from build123d import *

# Parameters (mm, degrees)
CROQUIS1_W              = 16
CROQUIS1_H              = 11.5
SALIENTE_EXTRUIR2_DEPTH = 8
CROQUIS3_W              = 14
CROQUIS3_H              = 9.5
CORTAR_EXTRUIR2_DEPTH   = 2
CROQUIS4_W              = 12
CROQUIS4_H              = 7.5
CORTAR_EXTRUIR3_DEPTH   = 5
REDONDEO1_R             = 1
REDONDEO2_R             = 0.5
CORTAR_EXTRUIR4_REACH   = 19.119
CROQUIS5_R              = 0.5
CORTAR_EXTRUIR5_REACH   = 16.773
CROQUIS6_R              = 0.5


with BuildPart() as part:
    # Croquis1 → Saliente-Extruir2 (new body)
    with BuildSketch(Plane(origin=(0, 0, 0), x_dir=(1, 0, 0), z_dir=(0, 1, 0))):
        Rectangle(CROQUIS1_W, CROQUIS1_H)
    extrude(amount=SALIENTE_EXTRUIR2_DEPTH)

    # Croquis3 → Cortar-Extruir2 (cut)
    with BuildSketch(Plane(origin=(0, 8, 0), x_dir=(1, 0, 0), z_dir=(0, 1, 0))):
        Rectangle(CROQUIS3_W, CROQUIS3_H)
    extrude(amount=-CORTAR_EXTRUIR2_DEPTH, mode=Mode.SUBTRACT)

    # Croquis4 → Cortar-Extruir3 (cut)
    with BuildSketch(Plane(origin=(0, 6, 0), x_dir=(1, 0, 0), z_dir=(0, 1, 0))):
        Rectangle(CROQUIS4_W, CROQUIS4_H)
    extrude(amount=-CORTAR_EXTRUIR3_DEPTH, mode=Mode.SUBTRACT)

    # Redondeo1
    redondeo1_edges = [part.edges().sort_by_distance(p)[0] for p in [
        (0, 0, 5.75),
        (8, 0, 0),
        (0, 0, -5.75),
        (-8, 0, 0),
        (-8, 4, 5.75),
        (8, 4, 5.75),
        (8, 4, -5.75),
        (-8, 4, -5.75),
    ]]
    fillet(redondeo1_edges, radius=REDONDEO1_R)

    # Redondeo2
    redondeo2_edges = [part.edges().sort_by_distance(p)[0] for p in [
        (7, 7, -4.75),
        (7, 7, 4.75),
        (-7, 7, 4.75),
        (-7, 7, -4.75),
    ]]
    fillet(redondeo2_edges, radius=REDONDEO2_R)

    # Croquis5 → Cortar-Extruir4 (cut, up to next)
    with BuildSketch(Plane.ZY.offset(-6), mode=Mode.PRIVATE) as cortar_extruir4_sk1:
        with Locations((-1.27, 3.5)):
            Circle(CROQUIS5_R)
    cortar_extruir4_tool1 = extrude(cortar_extruir4_sk1.sketch, amount=-CORTAR_EXTRUIR4_REACH, mode=Mode.PRIVATE) & part.part
    # Croquis5 → Cortar-Extruir4 (cut, up to next)
    with BuildSketch(Plane.ZY.offset(-6), mode=Mode.PRIVATE) as cortar_extruir4_sk2:
        with Locations((1.27, 3.5)):
            Circle(CROQUIS5_R)
    cortar_extruir4_tool2 = extrude(cortar_extruir4_sk2.sketch, amount=-CORTAR_EXTRUIR4_REACH, mode=Mode.PRIVATE) & part.part
    add(cortar_extruir4_tool1.solids().sort_by_distance((6, 3.5, -1.27))[0], mode=Mode.SUBTRACT)
    add(cortar_extruir4_tool2.solids().sort_by_distance((6, 3.5, 1.27))[0], mode=Mode.SUBTRACT)

    # Croquis6 → Cortar-Extruir5 (cut, up to next)
    with BuildSketch(Plane.XY.offset(-3.75), mode=Mode.PRIVATE) as cortar_extruir5_sk1:
        with Locations((1.905, 3.5)):
            Circle(CROQUIS6_R)
    cortar_extruir5_tool1 = extrude(cortar_extruir5_sk1.sketch, amount=-CORTAR_EXTRUIR5_REACH, mode=Mode.PRIVATE) & part.part
    # Croquis6 → Cortar-Extruir5 (cut, up to next)
    with BuildSketch(Plane.XY.offset(-3.75), mode=Mode.PRIVATE) as cortar_extruir5_sk2:
        with Locations((-1.905, 3.5)):
            Circle(CROQUIS6_R)
    cortar_extruir5_tool2 = extrude(cortar_extruir5_sk2.sketch, amount=-CORTAR_EXTRUIR5_REACH, mode=Mode.PRIVATE) & part.part
    add(cortar_extruir5_tool1.solids().sort_by_distance((1.905, 3.5, -3.75))[0], mode=Mode.SUBTRACT)
    add(cortar_extruir5_tool2.solids().sort_by_distance((-1.905, 3.5, -3.75))[0], mode=Mode.SUBTRACT)


solid = part.part
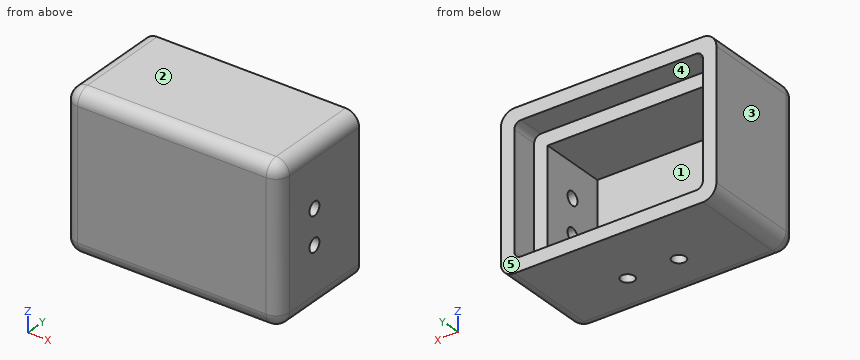
Geometry check sheet. Reference: the model listing, model coordinates, mm. Face numbers are marked on the shaded views. A direction names the side the tool comes from. Give positions to 0.01 mm unless a question says otherwise; leave off trailing zeros. Order: outer loops, then holes, each group sorted by start corner. A loop starts at its lowest first (then second) coordinate and runs counter-clockwise, first axis right, second up. Notation, with made-up numbers: M 74,-26.75 L 93,-26.75 A18 ccw 93,-10.75 Z; hole C -15.5,68 d6. An arc over 180 degrees is marked long. Use a Markdown table: item, result.
Item 1: Section check B-B (y = 1.5). Record the cut outline in (x, z).
Answers follow:
| item | result |
|---|---|
| outline | M -8,-4.75 A1 ccw -7,-5.75 L 7,-5.75 A1 ccw 8,-4.75 L 8,4.75 A1 ccw 7,5.75 L -7,5.75 A1 ccw -8,4.75 Z; hole M -6,-3.75 L 6,-3.75 L 6,3.75 L -6,3.75 Z |
Item 2: Section check D-D (x = -5.75). Record the cut outline in (y, z).
Answers follow:
| item | result |
|---|---|
| outline | M 0,-4.75 A1 ccw 1,-5.75 L 8,-5.75 L 8,-4.75 L 6,-4.75 L 6,-3.75 L 1,-3.75 L 1,3.75 L 6,3.75 L 6,4.75 L 8,4.75 L 8,5.75 L 1,5.75 A1 ccw 0,4.75 Z |
Item 3: Tool access check on the marked faces 1 and 2. Record the directions out of +Z, -Z, +X, -X, +Y, -Y that give a thin tool (end or side, any length) a straight path to the whole face; none if there is none.
Answers follow:
| item | result |
|---|---|
| face 1 | +Y |
| face 2 | +Z, +X, -X, +Y, -Y |
Item 4: Section check A-A (y = 3.5). Record the cut outline in (x, z) (3 decimals).
Answers follow:
| item | result |
|---|---|
| outline | M -8,-4.75 A1 ccw -7,-5.75 L -2.405,-5.75 L -2.405,-3.75 L -6,-3.75 L -6,3.75 L 6,3.75 L 6,1.77 L 8,1.77 L 8,4.75 A1 ccw 7,5.75 L -7,5.75 A1 ccw -8,4.75 Z; M -1.405,-5.75 L 1.405,-5.75 L 1.405,-3.75 L -1.405,-3.75 Z; M 2.405,-5.75 L 7,-5.75 A1 ccw 8,-4.75 L 8,-1.77 L 6,-1.77 L 6,-3.75 L 2.405,-3.75 Z; M 6,-0.77 L 8,-0.77 L 8,0.77 L 6,0.77 Z |
Item 5: Depth check by flat-ended pin: P1, Ø2, axis at x = -0.5, z = 1, coming from the +Y side. Enter the tip coordinate at first touch or a pass-through.
Answers follow:
| item | result |
|---|---|
| P1 | stops at y = 1 |
Item 6: Draft check along X on the marked faces 3, 4 and 5. Enter one of: +X half, -X half, draft (parallel to the pull), parting line (faces both ways), or undercut.
Answers follow:
| item | result |
|---|---|
| face 3 | -X half |
| face 4 | undercut |
| face 5 | draft |
Item 7: Material ranges on line 1 along Z through (x, y) = (-1, 4.25); line 2 along X through (y, z) = (3, 3); line 3 along X through (y, z) = (6.25, 3), recorded low to high.
Answers follow:
| item | result |
|---|---|
| line 1 | z = -5.75 to -3.75, 3.75 to 5.75 |
| line 2 | x = -8 to -6, 6 to 8 |
| line 3 | x = -8 to -7, 7 to 8 |
Item 8: Section check C-C (z = -1.27). Record the cut outline in (x, y).
Answers follow:
| item | result |
|---|---|
| outline | M -8,1 A1 ccw -7,0 L 7,0 A1 ccw 8,1 L 8,3 L 6,3 L 6,1 L -6,1 L -6,6 L -7,6 L -7,8 L -8,8 Z; M 6,4 L 8,4 L 8,8 L 7,8 L 7,6 L 6,6 Z |
